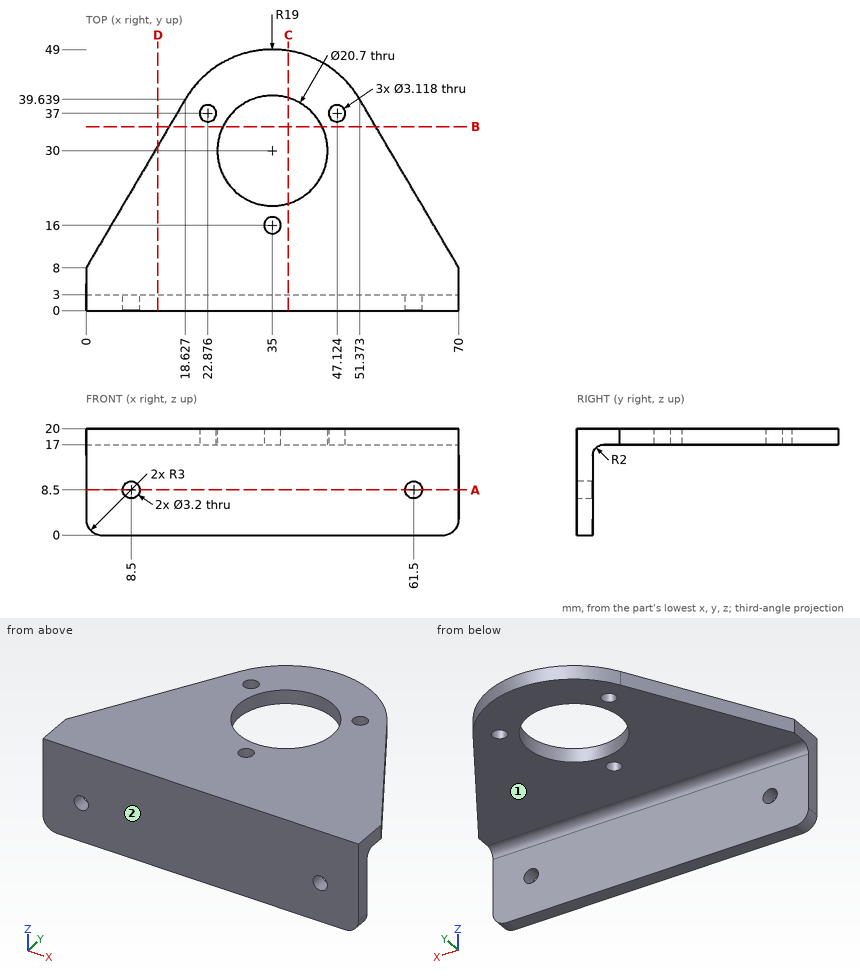
Here's the drawing with two shaded views (mm, measured from the low corner). I have some questions. A direction names the side the tool comes from. Give positions to 0.01 mm unless a question says otherwise; leave off trailing zeros. Order: outer loops, then holes, each group sorted by start corner. A loop starts at its lowest first (then second) coordinate and runs counter-clockwise, first axis right, second up. Notation, with made-up numbers: (16, 81.5) - (30, 81.5) arc R32 ccw to (30, 112.5) - close; hole circle Ø4 at (3, 53). An arc over 180 degrees is marked (long way). Use a Markdown table: item, result. Add a question column.
Q1. If we section it at A-A on z = 8.5: Write out the boundary of the cut face in (x, y), plus the area to 3 significant figures.
Q2. If we section it at D-D on x = 13.5: Write out the boundary of the cut face in (y, z).
Q3. Please list where these lines run through material, in increasing order: line 1 along X through (y, z) = (1.85, 8.5); line 2 along Y through (x, z) = (11.5, 13.5); line 3 along Z through (x, y) = (50, 10).
Q4. On a 3-axis mill with a long thin cutter (end or side, diameter ignored), from which of +Z, -Z, +X, -X, +Y, -Y can I reach the whole of each face in a straight line? I mean the marked faces 1 and 2. Say none if no direction works.
Q5. If we section it at C-C on x = 38: Write out the boundary of the cut face in (y, z) (1 decimal), plus the area to 3 significant figures.
Q6. If we section it at B-B on y = 34.5: Write out the boundary of the cut face in (x, z).
Q7. I'm going to push flat-ended pins straight in: pin 1 (2 mm diameter, centred on x = 48.5, y = 33.5, fed in from -Z); pin 2 (12 mm diameter, centred on x = 58.5, z = 5.5, fed in from +Y); pin 3 (10 mm diameter, centred on y = 32.5, z = 14.5, fed in from +X) (1 decimal); pin 4 (12.5 mm diameter, centred on x = 35, y = 30, fed in from -Z). Where does each tip first touch, or does it pass through?
Answers follow:
| question | item | result |
|---|---|---|
| 1 | outline | (0, 0) - (6.9, 0) - (6.9, 3) - (0, 3) - close; (10.1, 0) - (59.9, 0) - (59.9, 3) - (10.1, 3) - close; (63.1, 0) - (70, 0) - (70, 3) - (63.1, 3) - close |
| 1 | area | 191 mm^2 |
| 2 | outline | (0, 0) - (3, 0) - (3, 15) arc R2 cw to (5, 17) - (30.93, 17) - (30.93, 20) - (0, 20) - close |
| 3 | line 1 | x = 0 to 6.9, 10.1 to 59.9, 63.1 to 70 |
| 3 | line 2 | y = 0 to 3 |
| 3 | line 3 | z = 17 to 20 |
| 4 | face 1 | -Z, +X, -X, +Y |
| 4 | face 2 | +Z, -Z, +X, -X, -Y |
| 5 | outline | (0, 0) - (3, 0) - (3, 15) arc R2 cw to (5, 17) - (20.1, 17) - (20.1, 20) - (0, 20) - close; (39.9, 17) - (48.8, 17) - (48.8, 20) - (39.9, 20) - close |
| 5 | area | 139 mm^2 |
| 6 | outline | (15.6, 17) - (25.68, 17) - (25.68, 20) - (15.6, 20) - close; (44.32, 17) - (54.4, 17) - (54.4, 20) - (44.32, 20) - close |
| 7 | pin 1 | stops at z = 17 |
| 7 | pin 2 | stops at y = 3 |
| 7 | pin 3 | stops at x = 58.1 |
| 7 | pin 4 | passes through |
